```python
from build123d import *

# Parameters (mm, degrees)
CHAMFER_1_SIZE           = 2
CHAMFER_1_SIZE2          = 3.464101615
CHAMFER_2_SIZE           = 1.5
SKETCH_2_W               = 2
SKETCH_2_H               = 31
CUT_EXTRUDE_1_DEPTH      = 32.559467676
PATTERN_CIRCULAR_1_COUNT = 10
CHAMFER_3_SIZE           = 5
CHAMFER_4_SIZE           = 1


with BuildPart() as part:
    # 草图1 → 旋转1 (revolve)
    with BuildSketch(Plane.XY, mode=Mode.PRIVATE) as revolve_1_sk:
        Polygon((-2.5, 0), (-2.5, 10), (-4.75, 10), (-4.75, 14), (-14.5, 14), (-14.5, 28), (-20, 28), (-20, 22), (-17, 22), (-17, 7), (-6.5, 7), (-6.5, 6), (-4.5, 6), (-4.5, 0), align=None)
    revolve(revolve_1_sk.sketch.rotate(Axis((0, 0, 0), (0, 1, 0)), 270), axis=Axis((0, 0, 0), (0, 1, 0)))

    # 倒角1
    chamfer_1_edges = [part.edges().sort_by_distance(p)[0] for p in [
        (0, 28, 14.5),
    ]]
    chamfer_1_side = [part.faces().sort_by_distance(p)[0] for p in [
        (0, 21, 14.5),
    ]]
    chamfer(chamfer_1_edges, length=CHAMFER_1_SIZE, length2=CHAMFER_1_SIZE2, reference=chamfer_1_side[0])

    # 倒角2
    chamfer_2_edges = [part.edges().sort_by_distance(p)[0] for p in [
        (0, 28, 20),
    ]]
    chamfer(chamfer_2_edges, length=CHAMFER_2_SIZE)

    # 草图2 → 切除-拉伸1 (cut, through all)
    with BuildSketch(Plane(origin=(0, 14, 0), x_dir=(1, 0, 0), z_dir=(0, 1, 0))):
        Rectangle(SKETCH_2_W, SKETCH_2_H)
    cut_extrude_1 = extrude(amount=CUT_EXTRUDE_1_DEPTH, mode=Mode.SUBTRACT)

    # 阵列(圆周)1: 切除-拉伸1 ×10 about axis
    pattern_circular_1_axis = Axis((0, 0, 0), (0, 1, 0))
    for i in range(1, PATTERN_CIRCULAR_1_COUNT):
        add(cut_extrude_1.rotate(pattern_circular_1_axis, i * 360 / PATTERN_CIRCULAR_1_COUNT), mode=Mode.SUBTRACT)

    # 倒角3
    chamfer_3_edges = [part.edges().sort_by_distance(p)[0] for p in [
        (0, 7, 17),
    ]]
    chamfer(chamfer_3_edges, length=CHAMFER_3_SIZE)

    # 倒角4
    chamfer_4_edges = [part.edges().sort_by_distance(p)[0] for p in [
        (0, 0, 4.5),
    ]]
    chamfer(chamfer_4_edges, length=CHAMFER_4_SIZE)


solid = part.part
```
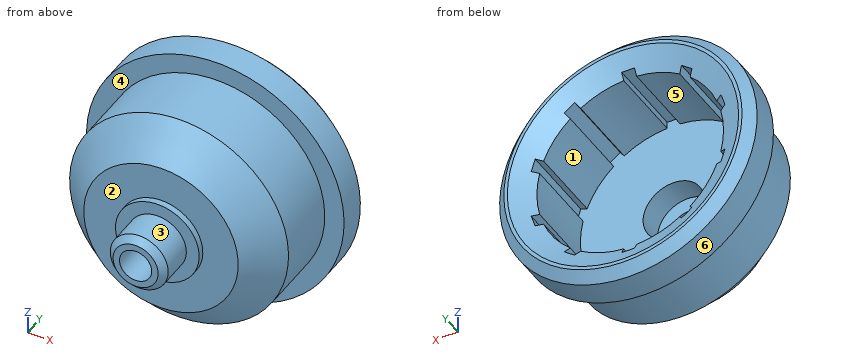
CAD build for the part. Positions are in the model's coordinates, mm. Face numbers are marked on the shaded views. A direction names the side the tool comes from. Give positions to 0.01 mm unless a question says otherwise; leave off trailing zeros. Loops run counter-clockwise (first coordinate to the right, second up) from the corner with the lowest first, then second, coordinate; pieces in that order, holes last. Notation, with made-up numbers: (31.25, 37.5) - (75.25, 37.5) arc R22 cw to (75.25, 53.5) - close; hole circle Ø5 at (85.5, 22). An arc over 180 degrees is marked (long way). Put each result on its own line as item: value.
Q1. Tool access for the marked faces 4, 5 and 6: list every direction of +Z, -Z, +X, -X, +Y, -Y with a clear straight run to the whole face (end or side of a thin tool).
Filled in:
face 4: -Y
face 5: +Y
face 6: +Y, -Y
Q2. Probe line 1 along X through (y, z) = (3.5, 0); line 2 along X through (y, z) = (12.1, 0); line 3 along Z through (x, y) = (1, 11). List the from-to ranges inside material, lowest first.
Filled in:
line 1: x = -4.5 to -2.5, 2.5 to 4.5
line 2: x = -17 to -4.75, 4.75 to 17
line 3: z = -15.97 to -4.64, 4.64 to 15.97
Q3. Mould opens along Z. For the marked faces 1, 2 and 3 say: pulls with the +Z half, pulls with the -Z half, needs draft (parallel to the pull), parting line crosses it, or undercut.
Filled in:
face 1: undercut
face 2: needs draft
face 3: parting line crosses it
Q4. Slice it at A-A (y = 3.75). Give the cut face in (x, z), plus the area to 3 significant figures.
Filled in:
outline: circle Ø9 at (0, 0); hole circle Ø5 at (0, 0)
area: 44.0 mm²
Q5. Flat gauge pins, fed straight in: pin 1 (24 mm diameter, centred on x = 3, z = 0, fed in from +Y); pin 2 (15 mm diameter, centred on x = 0, z = 0, fed in from +Y); pin 3 (1.5 mm diameter, centred on x = 15.5, z = 10, fed in from -Y). Where does each tip first touch, or does it go through?
Filled in:
pin 1: stops at y = 26.29
pin 2: stops at y = 14
pin 3: stops at y = 22
